```python
from build123d import *

# Parameters (mm, degrees)
F0_W     = 7.9375
F0_H     = 34.925
F1_DEPTH = 7.9375
F2_R     = 1.35255
F3_DEPTH = 6.35
F4_R     = 1.35255
F5_DEPTH = 6.35
F7_DEPTH = 7.9375


with BuildPart() as f1:
    # F0 (on Top) → F1 (new body)
    with BuildSketch(Plane.XY):
        Rectangle(F0_W, F0_H)
        with BuildLine():
            Line((1.5875, 3.175), (1.5875, -3.175))
            ThreePointArc((1.5875, -3.175), (0, -4.7625), (-1.5875, -3.175))
            Line((-1.5875, -3.175), (-1.5875, 3.175))
            ThreePointArc((-1.5875, 3.175), (0, 4.7625), (1.5875, 3.175))
        make_face(mode=Mode.SUBTRACT)
    extrude(amount=F1_DEPTH)

    # F2 (on face) → F3 (cut)
    with BuildSketch(Plane(origin=(0, 0, 0), x_dir=(1, 0, 0), z_dir=(0, 0, -1))):
        with Locations((0, -7.9375)):
            Circle(F2_R)
        with Locations((0, 7.9375)):
            Circle(F2_R)
    extrude(amount=-F3_DEPTH, mode=Mode.SUBTRACT)

    # F4 (on face) → F5 (cut)
    with BuildSketch(Plane.YZ.offset(3.96875)):
        with Locations((14.2875, 3.96875)):
            Circle(F4_R)
        with Locations((-14.2875, 3.96875)):
            Circle(F4_R)
    extrude(amount=-F5_DEPTH, mode=Mode.SUBTRACT)

    # F6 (on face) → F7 (cut, through all)
    with BuildSketch(Plane(origin=(-3.96875, 0, 0), x_dir=(0, -1, 0), z_dir=(-1, 0, 0))):
        with BuildLine():
            Line((-1.5875, 3.175), (-1.5875, 0))
            Line((-1.5875, 0), (1.5875, 0))
            Line((1.5875, 0), (1.5875, 3.175))
            ThreePointArc((1.5875, 3.175), (0, 4.7625), (-1.5875, 3.175))
        make_face()
    extrude(amount=-F7_DEPTH, mode=Mode.SUBTRACT)


solid = f1.part
```
The listing builds one solid part. Answer for the finished solid, in the listing's coordinates (mm). A direction names the side the tool comes from. Coordinates: 2 decimals unless noted, no trailing zeros. Loops run counter-clockwise (first coordinate to the right, second up) from the corner with the lowest first, then second, coordinate; pieces in that order, holes last. Notation, with made-up numbers: M -30,-1 L -25,-1 A13 cw -25,14 Z; hole C 54.5,7.5 d3. An arc over 180 degrees is marked long. Answer as a JSON object with one key per item and string values. Group by question number.
Item 1: Consider L1, parallel to Y at x = 0, z = 4; L2, parallel to X at y = -1, z = 5.75; L3, parallel to X at y = -8, z = 6. Determine where each line is inside the solid, lowest interval first.
Item 2: Section B-B (y = 0) is taken. Write down the section's boundary in (x, z).
Item 3: Each of these flat-tipped pins is pushed along its axis until it touches: P1, Ø2, axis at x = 0, y = -7.5, coming from the -Z side; P2, Ø2.5, axis at x = 0, y = 7.94, coming from the -Z side; P3, Ø1.4, axis at y = -14, z = 4.5, coming from the +X side. Where does it stop, or does it pass through?
Item 4: Determine the mould class of faces 1 (the face through (0.838, 15.537, 3.451)), 2 (the face through (1.588, 0, 5)), 3 (the face through (2, 0, 7.938)), 4 (the face through (0.84, -15.64, 4.03)) for opening direction Z: +Z half, -Z half, draft (parallel to the pull), parting line (faces both ways), or undercut.
Item 5: Which of the six approach directions +Z, -Z, +X, -X, +Y, -Y give full straight-line access (tool end or side, diameter ignored) to faces 5 (the face through (-3, -1.588, 2)), 6 (the face through (-2.381, 14, 4)), 7 (the face through (-0.2, 6.6, 3.1)), 8 (the face through (0, 10, 0)), 9 (the face through (0.035, -4.762, 3.913))?
Item 6: Section A-A (x = 0) is taken. Write down the section's boundary in (y, z), and give its area (3 significant figures).
Item 7: Section D-D (x = 3) is taken. Write down the section's boundary in (y, z) (1 decimal), and give its area (3 significant figures).
Item 8: Section C-C (z = 3.5) is taken. Write down the section's boundary in (x, y) (1 decimal).
Solved:
{
 "1": {"L1": "y = -17.46 to -15.64, -12.94 to -9.29, -6.58 to -4.76, 4.76 to 6.58, 9.29 to 12.94, 15.64 to 17.46", "L2": "x = -3.97 to -1.59, 1.59 to 3.97", "L3": "x = -3.97 to -1.35, 1.35 to 3.97"},
 "2": {"outline": "M -3.97,4.76 L -1.59,4.76 L -1.59,7.94 L -3.97,7.94 Z; M 1.59,4.76 L 3.97,4.76 L 3.97,7.94 L 1.59,7.94 Z"},
 "3": {"P1": "stops at z = 0", "P2": "stops at z = 6.35", "P3": "stops at x = -2.38"},
 "4": {"face 1": "undercut", "face 2": "draft", "face 3": "+Z half", "face 4": "undercut"},
 "5": {"face 5": "-Z, +X, -X", "face 6": "+X", "face 7": "-Z", "face 8": "-Z, +X, -X, +Y, -Y", "face 9": "+Z, -Z"},
 "6": {"outline": "M -17.46,0 L -9.29,0 L -9.29,6.35 L -6.58,6.35 L -6.58,0 L -4.76,0 L -4.76,7.94 L -17.46,7.94 Z; M 4.76,0 L 6.58,0 L 6.58,6.35 L 9.29,6.35 L 9.29,0 L 17.46,0 L 17.46,7.94 L 4.76,7.94 Z; hole C -14.29,3.97 d2.71; hole C 14.29,3.97 d2.71", "area": "156 mm2"},
 "7": {"outline": "M -17.5,0 L -1.6,0 L -1.6,3.2 A1.6 cw 1.6,3.2 L 1.6,0 L 17.5,0 L 17.5,7.9 L -17.5,7.9 Z; hole C -14.3,4 d2.7; hole C 14.3,4 d2.7", "area": "252 mm2"},
 "8": {"outline": "M -4,-17.5 L 4,-17.5 L 4,-15.6 L -2.4,-15.6 L -2.4,-13 L 4,-13 L 4,-1.6 L 1.6,-1.6 L 1.6,-3.2 A1.6 cw -1.6,-3.2 L -1.6,-1.6 L -4,-1.6 Z; M -4,1.6 L -1.6,1.6 L -1.6,3.2 A1.6 cw 1.6,3.2 L 1.6,1.6 L 4,1.6 L 4,13 L -2.4,13 L -2.4,15.6 L 4,15.6 L 4,17.5 L -4,17.5 Z; hole C 0,-7.9 d2.7; hole C 0,7.9 d2.7"}
}
